Part model, mm, in its own coordinate system. Face numbers are marked on the shaded views. A direction names the side the tool comes from. Coordinates: 2 decimals unless noted, no trailing zeros. Order: outer loops, then holes, each group sorted by start corner. A loop starts at its lowest first (then second) coordinate and runs counter-clockwise, first axis right, second up. Notation, with made-up numbers: M 35.5,-28.5 L 90.5,-28.5 A13 ccw 90.5,-19.5 Z; hole C 69.25,-18 d11. An arc over 180 degrees is marked long. Answer in a Markdown table with one row per item. Add a question column.
from build123d import *

# Parameters (mm, degrees)
EXTRUDE_1_DEPTH = 200
FILLET_1_R      = 14
SKETCH_2_W      = 2
SKETCH_2_H      = 200
EXTRUDE_2_DEPTH = 20


with BuildPart() as part:
    # 草圖1 → 填料-伸長1 (new body)
    with BuildSketch(Plane(origin=(0, 0, 0), x_dir=(1, 0, 0), z_dir=(0, 1, 0))):
        Polygon((-27.501723192, 6.859259259), (-23.001723192, 6.859259259), (-23.001723192, 2.359259259), (4.748276808, 2.359259259), (12.331610141, 9.942592593), (12.331610141, 22.359259259), (16.361610141, 22.359259259), (16.361610141, 9.942592593), (4.778276808, -1.640740741), (-35.251723192, -1.640740741), (-35.251723192, 2.359259259), (-27.501723192, 2.359259259), align=None)
    extrude(amount=EXTRUDE_1_DEPTH)

    # 圓角1
    fillet_1_edges = [part.edges().sort_by_distance(p)[0] for p in [
        (16.361610141, 100, -9.942592593),
        (4.778276808, 100, 1.640740741),
    ]]
    fillet(fillet_1_edges, radius=FILLET_1_R)

    # 草圖2 → 填料-伸長2 (add)
    with BuildSketch(Plane(origin=(0, 0, -2.359259259), x_dir=(-1, 0, 0), z_dir=(0, 0, -1))):
        with Locations((14.151723192, 100)):
            Rectangle(SKETCH_2_W, SKETCH_2_H)
    extrude(amount=EXTRUDE_2_DEPTH)


solid = part.part
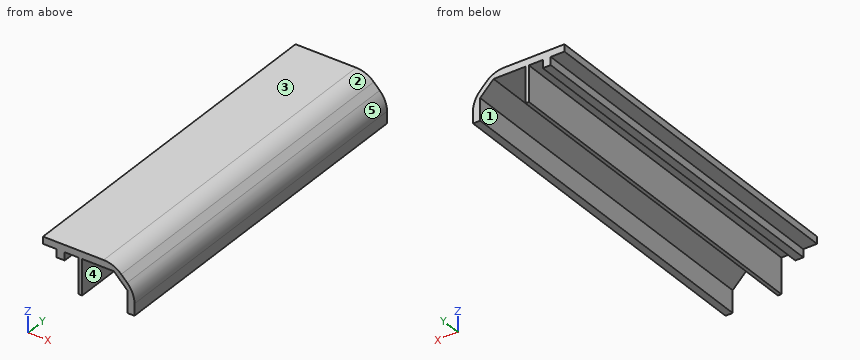
(1) Slice it at D-D (x = 2). List the corners of the cut face in (y, z).
(2) Drop flat-ended pins along their axis: P1, Ø1, axis at x = 2.5, y = 157, coming from the +Z side; P2, Ø1.5, axis at x = 0, y = 100.5, coming from the -Z side; P3, Ø3.5, axis at y = 95.5, z = -4.5, coming from the +X side. Give the stop position or say it passes through.
(3) Slice it at B-B (y = 118.5). List the corners of the cut face in (x, z).
(4) 3-axis set-ups, long thin cutter, end or side, ignore diameter. For the marked faces 4 and 5: which of +Z, -Z, +X, -X, +Y, -Y reach the whole face in a straight line?
(5) Slice it at C-C (x = -9.5). List the corners of the cut face in (y, z).
(6) Slice it at A-A (z = -12). List the corners of the cut face in (x, y).
(7) Pull direction X, two halves, no side cores. Call the marked faces 1, 2 and 3: pulls with the +X half, pulls with the -X half, needs draft (parallel to the pull), parting line crosses it, or undercut.
(8) Wall check: line 1 (X direction, y = 139, z = -20.5); line 2 (Z direction, x = -6.5, y = 79); line 3 (X direction, y = 118.5, z = -13). Give the ranges that are in metal, low to high.
Computed:
| question | item | result |
|---|---|---|
| 1 | outline | M 0,-2.36 L 200,-2.36 L 200,1.31 L 0,1.31 Z |
| 2 | P1 | stops at z = 1.31 |
| 2 | P2 | stops at z = -2.36 |
| 2 | P3 | stops at x = 12.65 |
| 3 | outline | M -35.25,-2.36 L -27.5,-2.36 L -27.5,-6.86 L -23,-6.86 L -23,-2.36 L -15.15,-2.36 L -15.15,-22.36 L -13.15,-22.36 L -13.15,-2.36 L 4.75,-2.36 L 12.33,-9.94 L 12.33,-22.36 L 16.36,-22.36 L 16.36,-15.74 A14 ccw 12.26,-5.84 L 8.88,-2.46 A14 ccw -1.02,1.64 L -35.25,1.64 Z |
| 4 | face 4 | -Z, +Y, -Y |
| 4 | face 5 | +Z, +X, +Y, -Y |
| 5 | outline | M 0,-2.36 L 200,-2.36 L 200,1.64 L 0,1.64 Z |
| 6 | outline | M -15.15,0 L -13.15,0 L -13.15,200 L -15.15,200 Z; M 12.33,0 L 15.85,0 L 15.85,200 L 12.33,200 Z |
| 7 | face 1 | undercut |
| 7 | face 2 | pulls with the +X half |
| 7 | face 3 | needs draft |
| 8 | line 1 | x = -15.15 to -13.15, 12.33 to 16.36 |
| 8 | line 2 | z = -2.36 to 1.64 |
| 8 | line 3 | x = -15.15 to -13.15, 12.33 to 16.09 |
